Read the model definition and answer for the solid it produces. Units are mm, in the model's axes. A direction names the side the tool comes from. Coordinates: 2 decimals unless noted, no trailing zeros. Order: outer loops, then holes, each group sorted by start corner. A loop starts at its lowest first (then second) coordinate and runs counter-clockwise, first axis right, second up. Notation, with made-up numbers: (22, 38.5) -> (26, 38.5) arc R10 cw to (26, 44.5) -> close; hole circle Ø3 at (-27.5, 51.5). An arc over 180 degrees is marked (long way). Answer in a Markdown table with one row per item.
from build123d import *

# Parameters (mm, degrees)
SKETCH1_R           = 4.5
BOSS_EXTRUDE1_DEPTH = 10
BOSS_EXTRUDE3_START = 4
SKETCH3_W           = 1.5
SKETCH3_H           = 1.5
BOSS_EXTRUDE3_DEPTH = 6


with BuildPart() as part:
    # Sketch1 → Boss-Extrude1 (new body)
    with BuildSketch(Plane.XY):
        Circle(SKETCH1_R)
        with BuildLine():
            Line((0.5, 2.958039892), (0.5, 3.5))
            Line((0.5, 3.5), (-0.5, 3.5))
            Line((-0.5, 3.5), (-0.5, 2.958039892))
            ThreePointArc((-0.5, 2.958039892), (0, -3), (0.5, 2.958039892))
        make_face(mode=Mode.SUBTRACT)
    extrude(amount=BOSS_EXTRUDE1_DEPTH)

    # Sketch3 → Boss-Extrude3 (add)
    with BuildSketch(Plane(origin=(0, 0, 0), x_dir=(1, 0, 0), z_dir=(0, 1, 0)).offset(BOSS_EXTRUDE3_START)):
        with Locations((0, -5)):
            Rectangle(SKETCH3_W, SKETCH3_H)
    extrude(amount=BOSS_EXTRUDE3_DEPTH)


solid = part.part
Q1. Given pin 1 (1.2 mm diameter, centred on x = 0, y = 6.5, fed in from -Z); pin 2 (1 mm diameter, centred on x = -2.5, z = 5.5, fed in from -Y); pin 3 (1.6 mm diameter, centred on y = 6, z = 4.5, fed in from +X), each flat-ended and moving along its own axis, determine where each tip first touches the part or whether it passes through.
Outcome:
| item | result |
|---|---|
| pin 1 | z = 4.25 |
| pin 2 | y = -4.03 |
| pin 3 | x = 0.75 |
Q2. Consider line 1 (Y direction, x = 0, z = 8); line 2 (Y direction, x = 0, z = 5.5); line 3 (X direction, y = -0.5, z = 4). Determine where each line is inside the solid, lowest interval first.
Outcome:
| item | result |
|---|---|
| line 1 | -4.5 to -3, 3.5 to 4.5 |
| line 2 | -4.5 to -3, 3.5 to 10 |
| line 3 | -4.47 to -2.96, 2.96 to 4.47 |
Q3. For faces 1 (the face through (-0.75, 7, 5)), 2 (the face through (0, 10, 5)), determine the directions among +Z, -Z, +X, -X, +Y, -Y from which every point of the face is accessible in a straight line to the end or side of a thin tool.
Outcome:
| item | result |
|---|---|
| face 1 | +Z, -Z, -X, +Y |
| face 2 | +Z, -Z, +X, -X, +Y |
Q4. The part is cut by section D-D (y = 2). Write down the section's boundary in (x, z), then the cut area to 3 significant figures.
Outcome:
| item | result |
|---|---|
| outline | (-4.03, 0) -> (-2.24, 0) -> (-2.24, 10) -> (-4.03, 10) -> close; (2.24, 0) -> (4.03, 0) -> (4.03, 10) -> (2.24, 10) -> close |
| area | 35.9 mm² |
Q5. The part is cut by section C-C (y = 0). Write down the section's boundary in (x, z).
Outcome:
| item | result |
|---|---|
| outline | (-4.5, 0) -> (-3, 0) -> (-3, 10) -> (-4.5, 10) -> close; (3, 0) -> (4.5, 0) -> (4.5, 10) -> (3, 10) -> close |
Q6. The part is cut by section B-B (z = 4.75). Write down the section's boundary in (x, y).
Outcome:
| item | result |
|---|---|
| outline | (-0.75, 4.44) arc R4.5 ccw (long way) to (0.75, 4.44) -> (0.75, 10) -> (-0.75, 10) -> close; hole (-0.5, 2.96) arc R3 ccw (long way) to (0.5, 2.96) -> (0.5, 3.5) -> (-0.5, 3.5) -> close |
Q7. For a pull along X with two mould halves and no side action, classify faces 3 (the face through (0, -3, 5)), 4 (the face through (1, -3, 10)), 5 (the face through (0, 3.5, 5)), 6 (the face through (0.75, 7, 5)) as pulls with the +X half, pulls with the -X half, needs draft (parallel to the pull), parting line crosses it, or undercut.
Outcome:
| item | result |
|---|---|
| face 3 | undercut |
| face 4 | needs draft |
| face 5 | undercut |
| face 6 | pulls with the +X half |
Q8. The part is cut by section A-A (x = 0). Write down the section's boundary in (y, z).
Outcome:
| item | result |
|---|---|
| outline | (-4.5, 0) -> (-3, 0) -> (-3, 10) -> (-4.5, 10) -> close; (3.5, 0) -> (4.5, 0) -> (4.5, 4.25) -> (10, 4.25) -> (10, 5.75) -> (4.5, 5.75) -> (4.5, 10) -> (3.5, 10) -> close |
